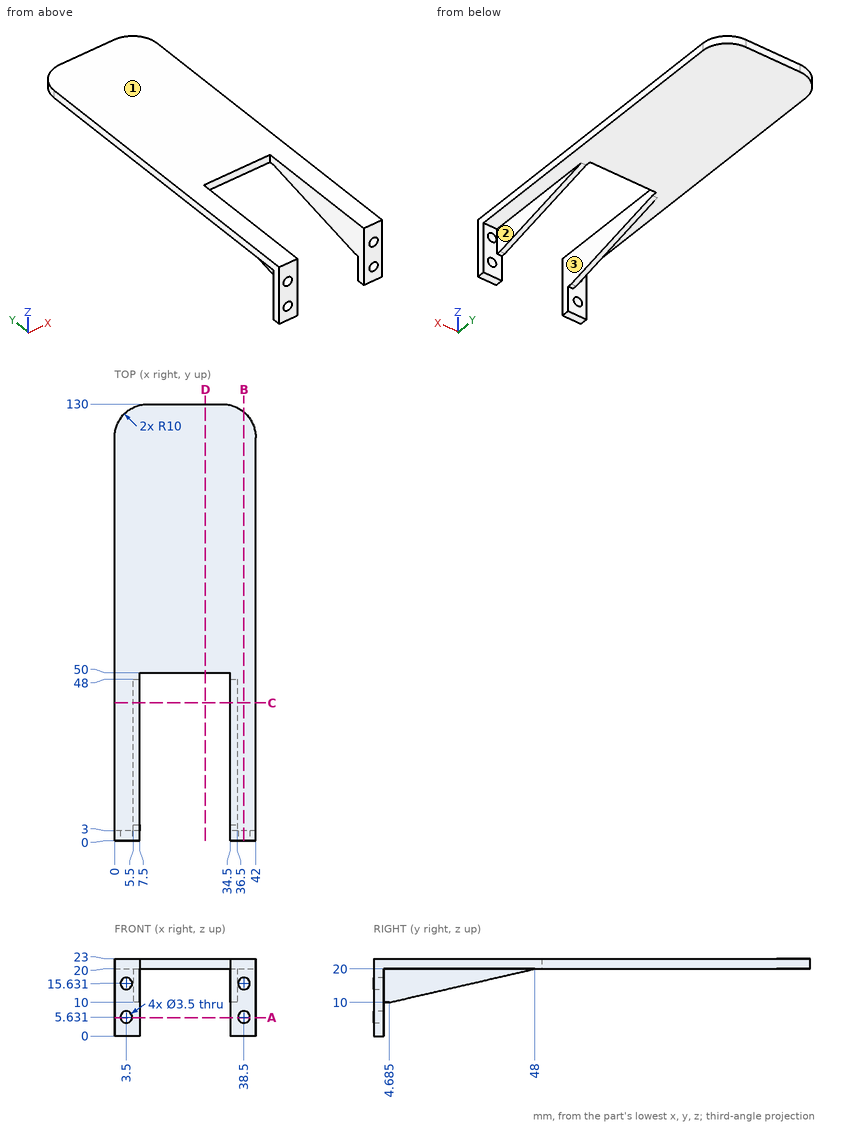
Answer from the drawing. Dimensions are ordinates in mm from the lowest x, y and z of the part. A direction names the side the tool comes from. Give positions to 0.01 mm unless a question says otherwise; leave off trailing zeros. Loops run counter-clockwise (first coordinate to the right, second up) from the corner with the lowest first, then second, coordinate; pieces in that order, holes last.
Item 1: For the marked faces 1, 2 and 3, determine the directions among +Z, -Z, +X, -X, +Y, -Y from which every point of the face is accessible in a straight line to the end or side of a thin tool.
Item 2: The part is cut by section A-A (z = 5.5). Write down the section's boundary in (x, y) (1 decimal).
Item 3: Each of these flat-tipped pins is pushed along its axis until it touches: pin 1 Ø2 at (x, z) = (39.5, 10.5) entering from +Y; pin 2 Ø7 at (y, z) = (24, 13) entering from +X; pin 3 Ø0.8 at (x, y) = (35.5, 3.5) entering from -Z; pin 4 Ø3 at (x, z) = (38.5, 15.63) entering from +Y. Where does it stop, or does it pass through?
Item 4: Find the intervals of material crossed by line 1 along Z through (x, y) = (3, 2) (1 decimal); line 2 along Y through (x, z) = (37, 3.5); line 3 along Z through (x, y) = (18, 68.5), in increasing order.
Item 5: The part is cut by section C-C (y = 41). Write down the section's boundary in (x, z).
Item 6: The part is cut by section D-D (x = 27). Write down the section's boundary in (y, z).
Item 7: The part is cut by section B-B (x = 38.5). Write down the section's boundary in (y, z).
Taken from the geometry:
1. face 1: +Z, +X, -X, +Y, -Y
1. face 2: -Z, +X, +Y
1. face 3: +Z, -Z, -Y
2. outline: (0, 0) - (1.8, 0) - (1.8, 3) - (0, 3) - close; (5.2, 0) - (7.5, 0) - (7.5, 3) - (5.2, 3) - close; (34.5, 0) - (36.8, 0) - (36.8, 3) - (34.5, 3) - close; (40.2, 0) - (42, 0) - (42, 3) - (40.2, 3) - close
3. pin 1: stops at y = 3
3. pin 2: stops at x = 36.5
3. pin 3: stops at z = 10
3. pin 4: passes through
4. line 1: z = 0 to 4, 7.3 to 14, 17.3 to 23
4. line 2: y = 0 to 3
4. line 3: z = 20 to 23
5. outline: (0, 20) - (5.5, 20) - (5.5, 18.38) - (7.5, 18.38) - (7.5, 23) - (0, 23) - close; (34.5, 18.38) - (36.5, 18.38) - (36.5, 20) - (42, 20) - (42, 23) - (34.5, 23) - close
6. outline: (50, 20) - (130, 20) - (130, 23) - (50, 23) - close
7. outline: (0, 0) - (3, 0) - (3, 3.88) - (0, 3.88) - close; (0, 7.38) - (3, 7.38) - (3, 13.88) - (0, 13.88) - close; (0, 17.38) - (3, 17.38) - (3, 20) - (127.6, 20) - (127.6, 23) - (0, 23) - close
